The drawing under review shows one solid part. Ordinate dimensions are in mm from its lowest x, y, z. Give positions to 0.01 mm unless a question says otherwise; leave off trailing zeros. Order: outer loops, then holes, each group sorted by start corner. A loop starts at its lowest first (then second) coordinate and runs counter-clockwise, first axis right, second up. Notation, with made-up numbers: M 8,-8 L 31,-8 A13 cw 31,16 Z; hole C 61,69 d9. An arc over 180 degrees is marked long. Put each result on its own line as item: value. Start each with the question number.
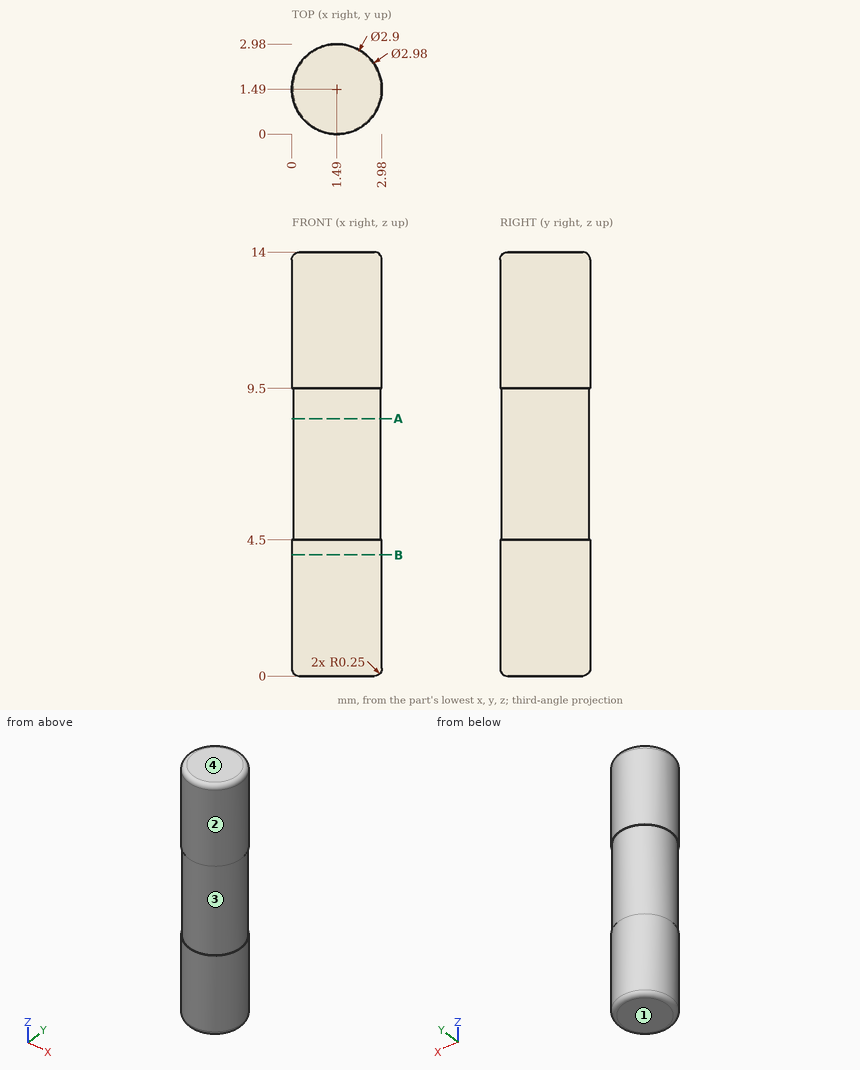
1. Insertion check: pin 1 (1.5 mm diameter, centred on x = 0.5, z = 10, fed in from +Y); pin 2 (1.5 mm diameter, centred on x = 2, z = 5.5, fed in from -Y); pin 3 (0.9 mm diameter, centred on x = 1, y = 2, fed in from -Z). Each pin has a flat end and moves straight along its axis. Give the tip position at first contact, or say it passes through.
2. The part is to be moulded in two halves that separate along Z. For the marked faces 1, 2, 3 and 4, say which applies: +Z half, -Z half, draft (parallel to the pull), parting line (faces both ways), or undercut.
3. Consider section B-B on z = 4. Give the boundary of the cut face in (x, y), then the cut area to 3 significant figures.
4. To check wall thickness, follow probe 1 along X at (y, z) = (1.65, 7); probe 2 along Y at (x, z) = (1.25, 7.75); probe 3 along Y at (x, z) = (1.15, 1.5). State the ranges of each line that lie inside material, in increasing order.
5. Consider section A-A on z = 8.5. Give the boundary of the cut face in (x, y), then the cut area to 3 significant figures.
Returned:
1. pin 1: stops at y = 2.96
1. pin 2: stops at y = 0.04
1. pin 3: stops at z = 0
2. face 1: -Z half
2. face 2: draft
2. face 3: undercut
2. face 4: +Z half
3. outline: C 1.49,1.49 d2.98
3. area: 6.97 mm2
4. probe 1: x = 0.05 to 2.93
4. probe 2: y = 0.06 to 2.92
4. probe 3: y = 0.04 to 2.94
5. outline: C 1.49,1.49 d2.9
5. area: 6.61 mm2
